```python
from build123d import *

# Parameters (mm, degrees)
PAD_DEPTH       = 60
POCKET_DEPTH    = 146.501
SKETCH002_W     = 132.291259
SKETCH002_H     = 95.159112
POCKET001_DEPTH = 5


with BuildPart() as part:
    # Sketch → Pad (new body, symmetric)
    with BuildSketch(Plane.XZ):
        with BuildLine():
            Line((-75.251187, 140.30381), (-47.669047, 6.945158))
            ThreePointArc((-47.669047, 6.945158), (-44.639819, 1.955924), (-39.140452, 0))
            Line((-39.140452, 0), (29.128963, 0))
            ThreePointArc((29.128963, 0), (32.06412, 1.215782), (33.279902, 4.150939))
            Line((33.279902, 4.150939), (33.279902, 32.237305))
            ThreePointArc((33.279902, 32.237305), (33.175099, 32.712971), (32.880098, 33.100547))
            Line((32.880098, 33.100547), (29.206815, 36.21552))
            ThreePointArc((31.147112, 38.503586), (29.032931, 38.329702), (29.206815, 36.21552))
            Line((31.147112, 38.503586), (35.845014, 34.519728))
            ThreePointArc((36.279902, 33.580735), (36.165902, 34.098141), (35.845014, 34.519728))
            Line((36.279902, 33.580735), (36.279902, 4.150939))
            ThreePointArc((29.128963, -3), (34.18544, -0.905538), (36.279902, 4.150939))
            Line((29.128963, -3), (-39.140452, -3))
            ThreePointArc((-50.606869, 6.337538), (-46.534171, -0.370324), (-39.140452, -3))
            Line((-50.606869, 6.337538), (-78.189009, 139.69619))
            ThreePointArc((-75.251187, 140.30381), (-77.023908, 141.468911), (-78.189009, 139.69619))
        make_face()
    extrude(amount=PAD_DEPTH, both=True)

    # Sketch001 → Pocket (cut, through all)
    with BuildSketch(Plane.XY.offset(-5)):
        Polygon((-30.454193, 45.645451), (-30.454193, -45.645451), (48.285122, -52.340881), (48.285122, 52.340881), align=None)
    extrude(amount=POCKET_DEPTH, mode=Mode.SUBTRACT)

    # Sketch002 (on Face7 of Pocket) → Pocket001 (cut)
    with BuildSketch(Plane(origin=(-44.336026, 0, -9.169877), x_dir=(-0.20254, 0, 0.979274), z_dir=(0.979274, 0, 0.20254))):
        with Locations((97.820296, 0)):
            Rectangle(SKETCH002_W, SKETCH002_H)
    extrude(amount=-POCKET001_DEPTH, mode=Mode.SUBTRACT)


solid = part.part
```
Read the model definition and answer for the solid it produces. Units are mm, in the model's axes. A direction names the side the tool comes from. Coordinates: 2 decimals unless noted, no trailing zeros. Loops run counter-clockwise (first coordinate to the right, second up) from the corner with the lowest first, then second, coordinate; pieces in that order, holes last. Notation, with made-up numbers: (-12.5, -16) - (10.5, -16) arc R32 ccw to (10.5, 13) - close; hole circle Ø9 at (-36, 43.25). An arc over 180 degrees is marked (long way). Answer in a Markdown table with one row per item.
1. Which of the six approach directions +Z, -Z, +X, -X, +Y, -Y give full straight-line access (tool end or side, diameter ignored) to faces 1 (the face through (32.03, 55.29, 1.18)), 2 (the face through (12.955, 49.337, -0.772)), 3 (the face through (-33, -5, -3))?
Conclusion:
| item | result |
|---|---|
| face 1 | +Y, -Y |
| face 2 | +Z, -Z, +X |
| face 3 | -Z, +X, -X, +Y, -Y |
2. Find section C-C, the plane z = 18.5. Write down the section's boundary in (x, y).
Conclusion:
| item | result |
|---|---|
| outline | (-53.12, -60) - (-50.06, -60) - (-50.06, 60) - (-53.12, 60) - close; (33.28, -60) - (36.28, -60) - (36.28, -51.32) - (33.28, -51.06) - close; (33.28, 51.06) - (36.28, 51.32) - (36.28, 60) - (33.28, 60) - close |
3. Find section D-D, the plane z = 107. Write down the section's boundary in (x, y).
Conclusion:
| item | result |
|---|---|
| outline | (-71.43, -60) - (-68.36, -60) - (-68.36, -47.58) - (-71.43, -47.58) - close; (-71.43, 47.58) - (-68.36, 47.58) - (-68.36, 60) - (-71.43, 60) - close |
4. Determine the mould class of faces 4 (the face through (-64, 47.58, 81)), 5 (the face through (-59, 60, 54)), 6 (the face through (12.64, -49.31, -0.77)), 7 (the face through (-33, 0, 0)) for opening direction Y: +Y half, -Y half, draft (parallel to the pull), parting line (faces both ways), or undercut.
Conclusion:
| item | result |
|---|---|
| face 4 | undercut |
| face 5 | +Y half |
| face 6 | undercut |
| face 7 | draft |
5. Find section B-B, the plane y = -13. Write down the section's boundary in (x, z).
Conclusion:
| item | result |
|---|---|
| outline | (-53.69, 21.24) - (-50.61, 6.34) arc R11.71 ccw to (-39.14, -3) - (-30.45, -3) - (-30.45, 0) - (-39.14, 0) arc R8.71 cw to (-47.67, 6.95) - (-50.75, 21.85) - close |
6. Given pin 1 (0.9 mm diameter, centred on y = 6, z = -1, fed in from +X); pin 2 (4.5 mm diameter, centred on y = -57.5, z = 25, fed in from -X); pin 3 (7 mm diameter, centred on y = 57, z = 20, fed in from -X), each flat-ended and moving along its own axis, determine where each tip first touches the part or whether it passes through.
Conclusion:
| item | result |
|---|---|
| pin 1 | stops at x = -30.45 |
| pin 2 | stops at x = -54.93 |
| pin 3 | stops at x = -54.16 |
7. Straight lines are drawn through the part: line 1 (Z direction, x = -37.5, y = 36.5); line 2 (X direction, y = -4, z = 12); line 3 (X direction, y = -10, z = 8). For each, find the intervals that lie inside material, in ascending order.
Conclusion:
| item | result |
|---|---|
| line 1 | z = -3 to 0 |
| line 2 | x = -51.78 to -48.71 |
| line 3 | x = -50.95 to -47.89 |
8. Find section A-A, the plane x = -7. Write down the section's boundary in (y, z).
Conclusion:
| item | result |
|---|---|
| outline | (-60, -3) - (-47.64, -3) - (-47.64, 0) - (-60, 0) - close; (47.64, -3) - (60, -3) - (60, 0) - (47.64, 0) - close |
